```python
from build123d import *

# Parameters (mm, degrees)
EXTRUDE_3_DEPTH     = 2
SKETCH_5_R          = 1
CUT_EXTRUDE_3_DEPTH = 2
SKETCH_6_W          = 20
SKETCH_6_H          = 55
EXTRUDE_4_DEPTH     = 2
EXTRUDE_5_DEPTH     = 2
SKETCH_9_R          = 1
CUT_EXTRUDE_4_DEPTH = 2
SKETCH_10_R         = 1
CUT_EXTRUDE_5_DEPTH = 2


with BuildPart() as part:
    # 草图3 → 凸台-拉伸3 (new body)
    with BuildSketch(Plane(origin=(0, 25.5, 0), x_dir=(-1, 0, 0), z_dir=(0, -1, 0))):
        Polygon((0, 37.906440796), (-13.266709079, 32.054566719), (-13.266709079, 5.851874077), (0, 0), (64, 0), (132.293984031, -27.379269049), (142.434829102, -10.14084507), (64, 36), align=None)
    extrude(amount=EXTRUDE_3_DEPTH)

    # 草图5 → 切除-拉伸3 (cut)
    with BuildSketch(Plane(origin=(0, 25.5, 0), x_dir=(-1, 0, 0), z_dir=(0, -1, 0))):
        with Locations((4.433290921, 18.953220398)):
            Circle(SKETCH_5_R)
    extrude(amount=CUT_EXTRUDE_3_DEPTH, mode=Mode.SUBTRACT)

    # 草图6 → 凸台-拉伸4 (add)
    with BuildSketch(Plane(origin=(-110.247854089, 0, 64.855488475), x_dir=(0.507042254, 0, 0.861921199), z_dir=(-0.861921199, 0, 0.507042254))):
        with Locations((-53.479867386, -2)):
            Rectangle(SKETCH_6_W, SKETCH_6_H)
    extrude(amount=-EXTRUDE_4_DEPTH)

    # 草图8 → 凸台-拉伸5 (add)
    with BuildSketch(Plane.XZ.offset(29.5)):
        Polygon((0, 0), (-64, 0), (-132.293984031, 27.379269049), (-142.434829102, 10.14084507), (-64, -36), (0, -37.906440796), (13.266709079, -32.054566719), (13.266709079, -5.851874077), align=None)
    extrude(amount=-EXTRUDE_5_DEPTH)

    # 草图9 → 切除-拉伸4 (cut)
    with BuildSketch(Plane.XZ.offset(29.5)):
        with Locations((-4.433290921, -18.953220398)):
            Circle(SKETCH_9_R)
    extrude(amount=-CUT_EXTRUDE_4_DEPTH, mode=Mode.SUBTRACT)

    # 草图10 → 切除-拉伸5 (cut)
    with BuildSketch(Plane(origin=(-110.247854089, 0, 64.855488475), x_dir=(0.507042254, 0, 0.861921199), z_dir=(-0.861921199, 0, 0.507042254))):
        with Locations((-53.479867386, -2)):
            Circle(SKETCH_10_R)
    extrude(amount=-CUT_EXTRUDE_5_DEPTH, mode=Mode.SUBTRACT)


solid = part.part
```
Verification items for the finished model (mm, model axes). Coordinates: 2 decimals unless noted, no trailing zeros. Write each loop counter-clockwise with the first axis right and the second up, starting at its lowest first coordinate (ties: lowest second). Pieces come first, ordered by that corner, then holes. Notation, with made-up numbers: M -20,6.5 L -15,6.5 A26 cw -15,29.5 Z; hole C 56,1 d8. An arc over 180 degrees is marked long. Answer as a JSON object with one key per item and string values. Group by question number.
(1) Release check for a two-part mould opening along Y. For faces 1 (the face through (-134.585, -1.643, 19.541)), 2 (the face through (6.73, -28.51, -2.97)), 3 (the face through (-63, 25.5, -13)) record: +Y half, -Y half, draft (parallel to the pull), parting line (faces both ways), or undercut.
(2) Cross-section at C-C, the plane z = 12. Record the cut outline in (x, y), and give its area (3 significant figures).
(3) Cross-section at A-A, the plane x = -76.5. Record the cut outline in (y, z), and give its area (3 significant figures).
(4) Cross-section at D-D, the plane y = 2. Record the cut outline in (x, z), and give its area (3 significant figures).
(5) Cross-section at B-B, the plane z = -3.5. Record the cut outline in (x, y).
(6) Gauge pin test, flat ends, axial feed: pin 1 (1.2 mm diameter, centred on x = -4.43, z = -18.95, fed in from -Y); pin 2 (2 mm diameter, centred on x = -45, y = -28.5, fed in from +Z). Record the tip position at first contact, or that the pin passes through.
(7) Material ranges on line 1 (Y direction, x = -13, z = -18.5); line 2 (X direction, y = 8, z = 15); line 3 (X direction, y = -23.5, z = 23), recorded low to high.
Reply:
{
 "1": {"face 1": "undercut", "face 2": "draft", "face 3": "+Y half"},
 "2": {"outline": "M -141.34,-29.5 L -93.93,-29.5 L -93.93,-27.5 L -139.02,-27.5 L -139.02,23.5 L -93.93,23.5 L -93.93,25.5 L -141.34,25.5 Z", "area": "308 mm²"},
 "3": {"outline": "M -29.5,-28.65 L -27.5,-28.65 L -27.5,5.01 L -29.5,5.01 Z; M 23.5,-28.65 L 25.5,-28.65 L 25.5,5.01 L 23.5,5.01 Z", "area": "135 mm²"},
 "4": {"outline": "M -142.43,10.14 L -140.71,9.13 L -130.57,26.37 L -132.29,27.38 Z", "area": "40.0 mm²"},
 "5": {"outline": "M -119.25,-29.5 L 7.93,-29.5 L 7.93,-27.5 L -119.25,-27.5 Z; M -119.25,23.5 L 7.93,23.5 L 7.93,25.5 L -119.25,25.5 Z"},
 "6": {"pin 1": "through", "pin 2": "z = 0"},
 "7": {"line 1": "-29.5 to -27.5, 23.5 to 25.5", "line 2": "-139.58 to -137.26", "line 3": "-134.87 to -132.55"}
}
